Verification items for the finished model (mm, model axes). A direction names the side the tool comes from. Round coordinates to 2 decimals unless told otherwise and drop trailing zeros. Order: outer loops, then holes, each group sorted by start corner. A loop starts at its lowest first (then second) coordinate and runs counter-clockwise, first axis right, second up. Notation, with made-up numbers: M 88.5,-39.5 L 123.5,-39.5 A12 cw 123.5,-33.5 Z; hole C -20.75,-9.5 d4. An arc over 180 degrees is marked long. Use one line per item in the form item = value. Start each with the question number.
Item 1: Cross-section at D-D on x = -7. Enter the section's corners in (y, z).
Item 2: Go/stop test with flat-tipped pins: pin 1 Ø2 at (x, z) = (26, 2.5) entering from +Y; pin 2 Ø2 at (y, z) = (10.5, 2.5) entering from +X; pin 3 Ø1.2 at (y, z) = (10, 2) entering from -X. Record where each tip stops, or that it passes through.
Item 3: Cross-section at C-C on z = 2.55. Enter the section's corners in (x, y).
Item 4: Tool access check on faces 1 (the flat face through (25, 5.5, 2)), 2 (the flat face through (-13.244, 10, 2)), 3 (the flat face through (16.756, 8, 2)), 4 (the flat face through (4, -5, 0)). Record the directions out of +Z, -Z, +X, -X, +Y, -Y that give a thin tool (end or side, any length) a straight path to the whole face; none if there is none.
Item 5: Cross-section at A-A on x = 4. Enter the section's corners in (y, z).
Item 6: Thickness scan on probe 1 along Y at (x, z) = (13, 1.3); probe 2 along Y at (x, z) = (-3, 3.15); probe 3 along Y at (x, z) = (4, 3.75). Record the ranges inside material, lowest first. Write a range as [from, to].
Item 7: Cross-section at B-B on y = -14. Enter the section's corners in (x, z), then the cut area to 3 significant figures.
Item 8: Release check for a two-part mould opening along Y. For faces 5 (the flat face through (5, 14.5, 2)), 6 (the flat face through (4, 9.5, 2)), 7 (the flat face through (28.256, -10, 2)) record: +Y half, -Y half, draft (parallel to the pull), parting line (faces both ways), or undercut.
from build123d import *

# Parameters (mm, degrees)
SKICA1_R                = 7.62
P_IDAT_VYSUNUT_M1_DEPTH = 4


with BuildPart() as part:
    # Skica1 → Přidat vysunutím1 (new body)
    with BuildSketch(Plane.XY):
        Polygon((-13.243861265, 5.499663067), (-19.743861265, 5.499663067), (-19.743861265, -24.500336933), (28.256138735, -24.500336933), (28.256138735, 5.499663067), (21.756138735, 5.499663067), (16.756138735, 5.499663067), (-8.243861265, 5.499663067), align=None)
        with Locations((-7.173861265, -12.250168466)):
            Circle(SKICA1_R, mode=Mode.SUBTRACT)
        with Locations((15.683146952, -11.880336933)):
            Circle(SKICA1_R, mode=Mode.SUBTRACT)
        Polygon((-13.243861265, 14.499663067), (-13.243861265, 5.499663067), (-8.243861265, 5.499663067), (-8.243861265, 9.499663067), (16.756138735, 9.499663067), (16.756138735, 5.499663067), (21.756138735, 5.499663067), (21.756138735, 14.499663067), align=None)
    extrude(amount=P_IDAT_VYSUNUT_M1_DEPTH)


solid = part.part
Output values:
q1.outline = M -24.5,0 L -19.87,0 L -19.87,4 L -24.5,4 Z; M -4.63,0 L 5.5,0 L 5.5,4 L -4.63,4 Z; M 9.5,0 L 14.5,0 L 14.5,4 L 9.5,4 Z
q2.pin_1 = 5.5
q2.pin_2 = 21.76
q2.pin_3 = -13.24
q3.outline = M -19.74,-24.5 L 28.26,-24.5 L 28.26,5.5 L 21.76,5.5 L 21.76,14.5 L -13.24,14.5 L -13.24,5.5 L -19.74,5.5 Z; hole C -7.17,-12.25 d15.24; hole M -8.24,5.5 L 16.76,5.5 L 16.76,9.5 L -8.24,9.5 Z; hole C 15.68,-11.88 d15.24
q4.face_1 = +Z, -Z, +X, +Y
q4.face_2 = +Z, -Z, -X, +Y
q4.face_3 = +Z, -Z
q4.face_4 = -Z, +X, -X, +Y, -Y
q5.outline = M -24.5,0 L 5.5,0 L 5.5,4 L -24.5,4 Z; M 9.5,0 L 14.5,0 L 14.5,4 L 9.5,4 Z
q6.probe_1 = [-24.5, -19.01], [-4.75, 5.5], [9.5, 14.5]
q6.probe_2 = [-24.5, -18.63], [-5.87, 5.5], [9.5, 14.5]
q6.probe_3 = [-24.5, 5.5], [9.5, 14.5]
q7.outline = M -19.74,0 L -14.59,0 L -14.59,4 L -19.74,4 Z; M 0.24,0 L 8.36,0 L 8.36,4 L 0.24,4 Z; M 23,0 L 28.26,0 L 28.26,4 L 23,4 Z
q7.area = 74.1 mm2
q8.face_5 = +Y half
q8.face_6 = undercut
q8.face_7 = draft
